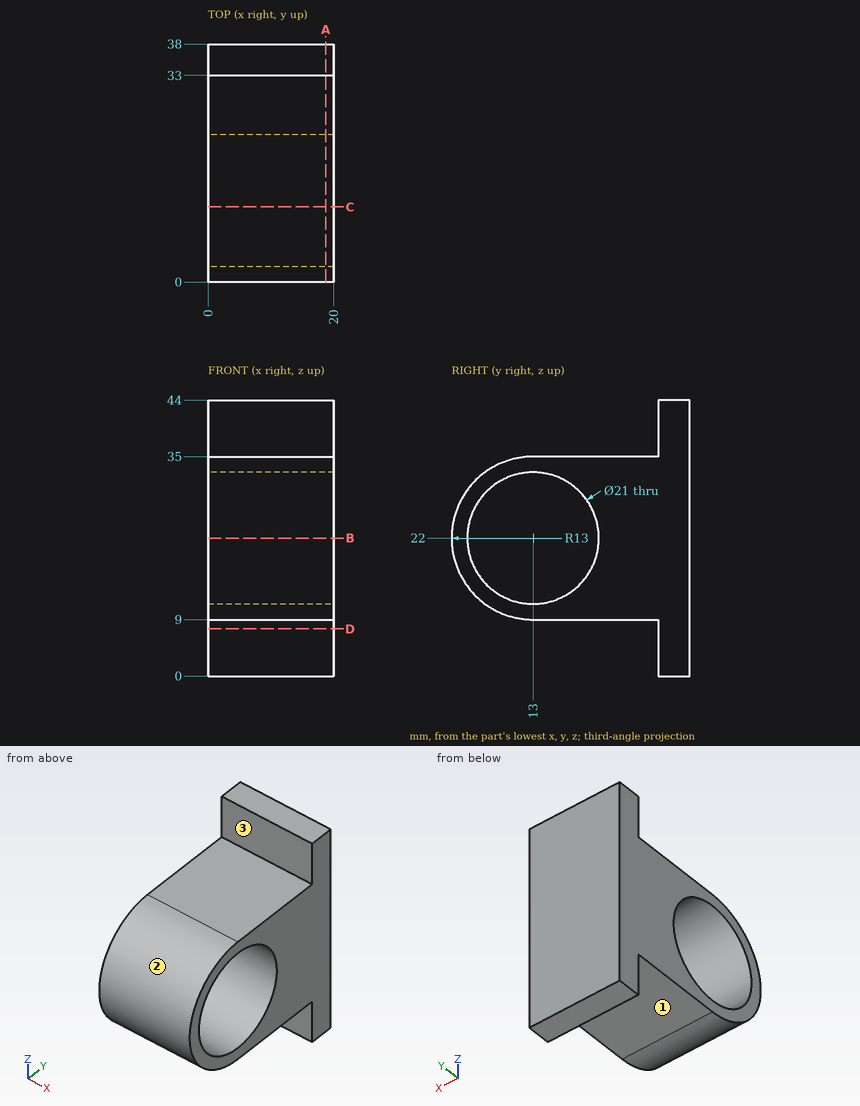
Design review of the part shown in the three views and the two pictorial views. Dimensions are in mm from the part's minimum x, y and z. A direction names the side the tool comes from. Round coordinates to 2 decimals unless told otherwise and drop trailing zeros. Loops run counter-clockwise (first coordinate to the right, second up) from the corner with the lowest first, then second, coordinate; pieces in that order, holes last.
Q1. To check wall thickness, follow line 1 along Y through (x, z) = (9.25, 22); line 2 along Z through (x, y) = (8.5, 21); line 3 along Y through (x, z) = (4.25, 17). State the ranges of each line that lie inside material, in increasing order.
Result sheet:
line 1: y = 0 to 2.5, 23.5 to 38
line 2: z = 9 to 15.2, 28.8 to 35
line 3: y = 1 to 3.77, 22.23 to 38
Q2. Machinability: for the marked faces 1, 2 and 3, which of the approach directions +Z, -Z, +X, -X, +Y, -Y give a long, thin tool a straight path to every point of the face, cutting with its end or side? Answer none if there is none.
Result sheet:
face 1: -Z, +X, -X, -Y
face 2: +X, -X, -Y
face 3: +Z, +X, -X, -Y
Q3. Insertion check: pin 1 Ø3 at (x, y) = (7, 27.5) entering from +Z; pin 2 Ø4 at (x, y) = (9.5, 30.5) entering from -Z; pin 3 Ø10 at (x, z) = (11, 38.5) entering from -Y. Each pin has a flat end and moves straight along its axis. Give the tip position at first contact, or say it passes through.
Result sheet:
pin 1: stops at z = 35
pin 2: stops at z = 9
pin 3: stops at y = 6.94
Q4. Add section C-C on y = 12. Write out the cut boundary in (x, z), plus the area to 3 significant figures.
Result sheet:
outline: (0, 9.04) - (20, 9.04) - (20, 11.55) - (0, 11.55) - close; (0, 32.45) - (20, 32.45) - (20, 34.96) - (0, 34.96) - close
area: 100 mm2
Q5. Add section D-D on z = 7.5. Write out the cut boundary in (x, y).
Result sheet:
outline: (0, 33) - (20, 33) - (20, 38) - (0, 38) - close
Q6. Add section B-B on z = 22. Write out the cut boundary in (x, y).
Result sheet:
outline: (0, 0) - (20, 0) - (20, 2.5) - (0, 2.5) - close; (0, 23.5) - (20, 23.5) - (20, 38) - (0, 38) - close
Q7. Add section A-A on x = 18.75. Write out the cut boundary in (y, z).
Result sheet:
outline: (13, 9) - (33, 9) - (33, 0) - (38, 0) - (38, 44) - (33, 44) - (33, 35) - (13, 35) arc R13 ccw to start; hole circle Ø21 at (13, 22)
